The listing builds one solid part. Answer for the finished solid, in the listing's coordinates (mm). Face numbers are marked on the shaded views. Coordinates: 2 decimals unless noted, no trailing zeros. Order: outer loops, then holes, each group sorted by start corner. A loop starts at its lowest first (then second) coordinate and runs counter-clockwise, first axis right, second up. Notation, with made-up numbers: (-21, -27) -> (-11, -27) arc R32 cw to (-11, 3) -> close; hole circle Ø10 at (-36.75, -25). An arc over 180 degrees is marked (long way). One line per question, with ' | ' between items.
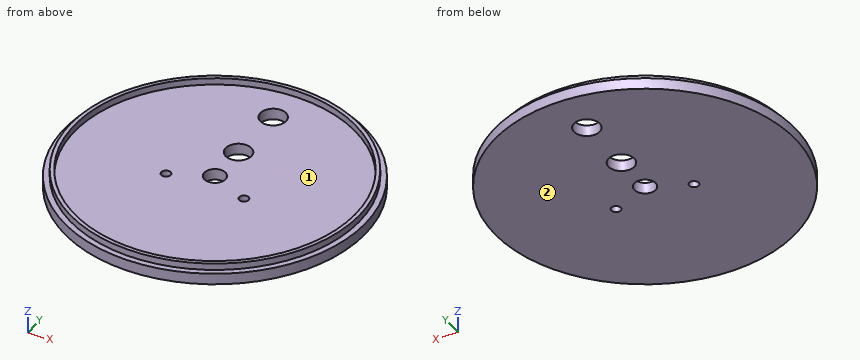
from build123d import *

# Parameters (mm, degrees)
F0_R      = 67
F1_DEPTH  = 5
F3_R      = 64.375
F3_R_2    = 62.625
F5_DEPTH  = 3
F7_R      = 2.1
F8_DEPTH  = 5.001
F6_R      = 5.75
F6_R_2    = 4.75
F9_DEPTH  = 5.001
F10_R     = 6.75
F10_R_2   = 5.75
F11_DEPTH = 0.5
F12_DEPTH = 0.5


with BuildPart() as f1:
    # F0 (on Top) → F1 (new body)
    with BuildSketch(Plane.XY):
        Circle(F0_R)
    extrude(amount=F1_DEPTH)

    # F3 (on face) → F5 (join)
    with BuildSketch(Plane.XY.offset(5)):
        Circle(F3_R)
        Circle(F3_R_2, mode=Mode.SUBTRACT)
    extrude(amount=F5_DEPTH)

    # F7 (on face) → F8 (cut, through all)
    with BuildSketch(Plane.XY.offset(5)):
        with Locations((17.4057390541, -7.9414527863)):
            Circle(F7_R)
        with Locations((-17.4057390541, -7.9414527863)):
            Circle(F7_R)
    extrude(amount=-F8_DEPTH, mode=Mode.SUBTRACT)

    # F6 (on face) → F9 (cut, through all)
    with BuildSketch(Plane.XY.offset(5)):
        with Locations((0, 46.25)):
            Circle(F6_R)
        with Locations((0, 18.75)):
            Circle(F6_R)
        Circle(F6_R_2)
    extrude(amount=-F9_DEPTH, mode=Mode.SUBTRACT)

    # F10 (on Top) → F11 (cut)
    with BuildSketch(Plane.XY):
        with Locations((0, 46.25)):
            Circle(F10_R)
        with Locations((0, 18.75)):
            Circle(F10_R)
        Circle(F10_R_2)
    extrude(amount=-F11_DEPTH, mode=Mode.SUBTRACT)

    # F10 (on Top) → F12 (cut)
    with BuildSketch(Plane.XY):
        with Locations((0, 46.25)):
            Circle(F10_R)
    extrude(amount=-F12_DEPTH, mode=Mode.SUBTRACT)


solid = f1.part
Item 1: Determine the mould class of the marked faces 1 and 2 for opening direction Y: pulls with the +Y half, pulls with the -Y half, needs draft (parallel to the pull), parting line crosses it, or undercut.
Computed values:
face 1: undercut | face 2: needs draft
Item 2: Section A-A, the plane y = 0 is taken. Give the vertices of the cut face in (x, z) (3 decimals).
Computed values:
outline: (-67, 0) -> (-4.75, 0) -> (-4.75, 5) -> (-62.625, 5) -> (-62.625, 8) -> (-64.375, 8) -> (-64.375, 5) -> (-67, 5) -> close; (4.75, 0) -> (67, 0) -> (67, 5) -> (64.375, 5) -> (64.375, 8) -> (62.625, 8) -> (62.625, 5) -> (4.75, 5) -> close
Item 3: Each of these flat-tipped pins is pushed along its axis until it touches: pin 1 Ø1 at (y, z) = (-31, 2) entering from +X; pin 2 Ø13 at (x, y) = (0, 18.75) entering from -Z; pin 3 Ø1 at (x, z) = (-37, 5) entering from +Y; pin 4 Ø6.5 at (x, y) = (-17.41, -7.94) entering from +Z. Where does it stop, or does it pass through?
Computed values:
pin 1: stops at x = 59.66 | pin 2: stops at z = 0 | pin 3: stops at y = 56.18 | pin 4: stops at z = 5
Item 4: Section D-D, the plane x = 37 is taken. Give the vertices of the cut face in (y, z).
Computed values:
outline: (-55.86, 0) -> (55.86, 0) -> (55.86, 5) -> (52.68, 5) -> (52.68, 8) -> (50.53, 8) -> (50.53, 5) -> (-50.53, 5) -> (-50.53, 8) -> (-52.68, 8) -> (-52.68, 5) -> (-55.86, 5) -> close
Item 5: Section B-B, the plane z = 3 is taken. Give the vertices of the cut face in (x, y).
Computed values:
outline: circle Ø134 at (0, 0); hole circle Ø4.2 at (-17.41, -7.94); hole circle Ø11.5 at (0, 18.75); hole circle Ø11.5 at (0, 46.25); hole circle Ø9.5 at (0, 0); hole circle Ø4.2 at (17.41, -7.94)
Item 6: Section C-C, the plane y = 46.25 is taken. Give the vertices of the cut face in (x, z).
Computed values:
outline: (-48.48, 0) -> (-5.75, 0) -> (-5.75, 5) -> (-42.22, 5) -> (-42.22, 8) -> (-44.78, 8) -> (-44.78, 5) -> (-48.48, 5) -> close; (5.75, 0) -> (48.48, 0) -> (48.48, 5) -> (44.78, 5) -> (44.78, 8) -> (42.22, 8) -> (42.22, 5) -> (5.75, 5) -> close
Item 7: Find the intervals of material crossed by L1, parallel to Y at x = 0, z = 1.7; L2, parallel to Y at x = 4, z = 6.75; L3, parallel to X at y = 22, z = 1.25, in increasing order.
Computed values:
L1: y = -67 to -4.75, 4.75 to 13, 24.5 to 40.5, 52 to 67 | L2: y = -64.25 to -62.5, 62.5 to 64.25 | L3: x = -63.29 to -4.74, 4.74 to 63.29
